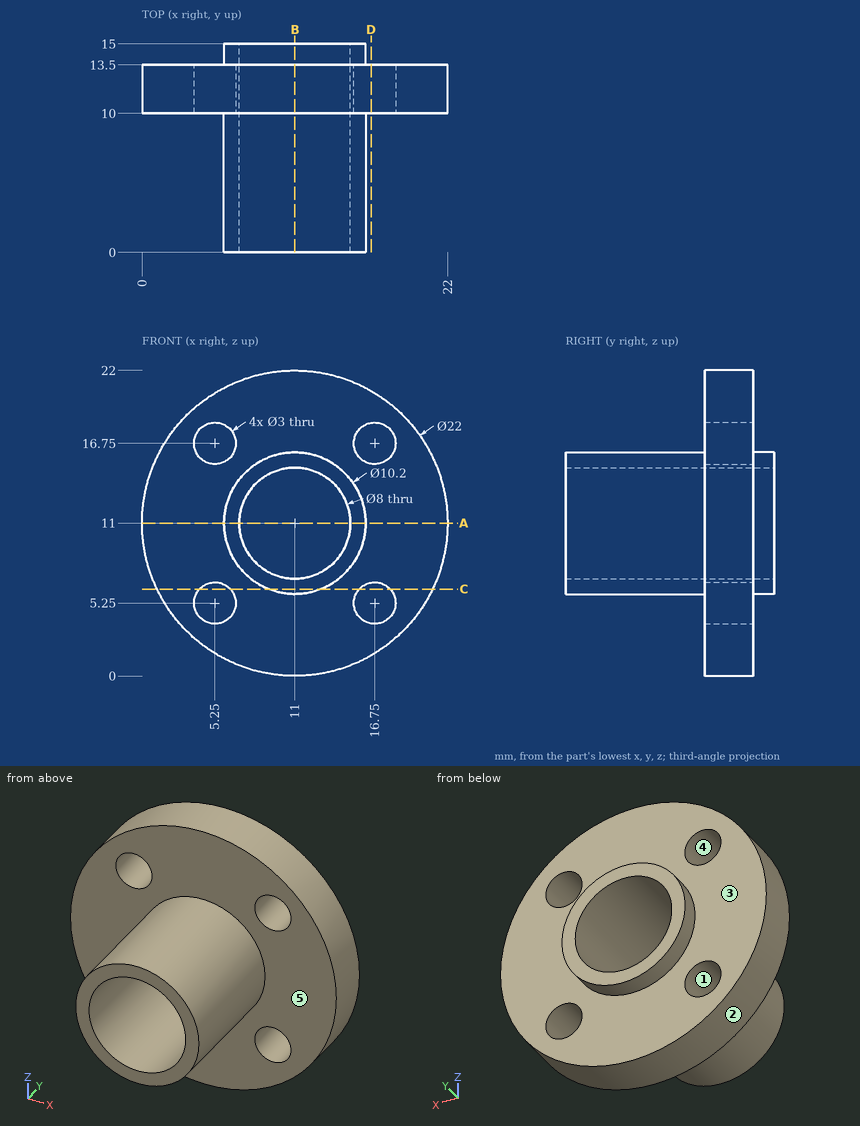
Design review of the part shown in the three views and the two pictorial views. Dimensions are in mm from the part's minimum x, y and z. A direction names the side the tool comes from. Round coordinates to 2 decimals unless told otherwise and drop trailing zeros. Order: outer loops, then holes, each group sorted by start corner. A loop starts at its lowest first (then second) coordinate and runs counter-clockwise, first axis right, second up.
Q1. We need section B-B, the plane x = 11. Give the boundary of the cut face in (y, z), plus the area to 3 significant figures.
Findings below:
outline: (0, 5.9) - (10, 5.9) - (10, 0) - (13.5, 0) - (13.5, 5.9) - (15, 5.9) - (15, 7) - (0, 7) - close; (0, 15) - (15, 15) - (15, 16.1) - (13.5, 16.1) - (13.5, 22) - (10, 22) - (10, 16.1) - (0, 16.1) - close
area: 74.3 mm2
Q2. Wall thickness on line 1 (Z direction, x = 5.25, y = 11.95); line 2 (Y direction, x = 18, z = 7.75): over which ranges is each line inside the solid? List them lowest first.
Findings below:
line 1: z = 1.62 to 3.75, 6.75 to 15.25, 18.25 to 20.38
line 2: y = 10 to 13.5
Q3. We need section A-A, the plane z = 11. Give the boundary of the cut face in (x, y).
Findings below:
outline: (0, 10) - (5.9, 10) - (5.9, 0) - (7, 0) - (7, 15) - (5.9, 15) - (5.9, 13.5) - (0, 13.5) - close; (15, 0) - (16.1, 0) - (16.1, 10) - (22, 10) - (22, 13.5) - (16.1, 13.5) - (16.1, 15) - (15, 15) - close
Q4. Machinability: for the marked faces 4 and 5, which of the approach directions +Z, -Z, +X, -X, +Y, -Y give a long, thin tool a straight path to every point of the face, cutting with its end or side? Answer none if there is none.
Findings below:
face 4: +Y, -Y
face 5: -Y
Q5. We need section D-D, the plane x = 16.5. Give the boundary of the cut face in (y, z), plus the area to 3 significant figures.
Findings below:
outline: (10, 1.47) - (13.5, 1.47) - (13.5, 3.77) - (10, 3.77) - close; (10, 6.73) - (13.5, 6.73) - (13.5, 15.27) - (10, 15.27) - close; (10, 18.23) - (13.5, 18.23) - (13.5, 20.53) - (10, 20.53) - close
area: 46.0 mm2
Q6. We need section C-C, the plane z = 6.25. Give the boundary of the cut face in (x, y).
Findings below:
outline: (1.08, 10) - (4.13, 10) - (4.13, 13.5) - (1.08, 13.5) - close; (6.37, 10) - (9.14, 10) - (9.14, 0) - (12.86, 0) - (12.86, 10) - (15.63, 10) - (15.63, 13.5) - (12.86, 13.5) - (12.86, 15) - (9.14, 15) - (9.14, 13.5) - (6.37, 13.5) - close; (17.87, 10) - (20.92, 10) - (20.92, 13.5) - (17.87, 13.5) - close
Q7. Mouldability with a two-part tool opening along X and no side actions: class the marked faces 1, 2 and 3 as pulls with the +X half, pulls with the -X half, needs draft (parallel to the pull), parting line crosses it, or undercut.
Findings below:
face 1: undercut
face 2: parting line crosses it
face 3: needs draft
Q8. Insertion check: P1, Ø1.8, axis at x = 5.25, z = 5.25, coming from the -Y side; P2, Ø6, axis at x = 8.5, y = 12, coming from the +Z side; P3, Ø5, axis at x = 16.75, z = 16.75, coming from the +Y side; P4, Ø3, axis at x = 8.5, y = 3.5, coming from the -Z side. Each pin has a flat end and moves straight along its axis. Give the tip position at first contact, or say it passes through.
Findings below:
P1: passes through
P2: stops at z = 22
P3: stops at y = 13.5
P4: stops at z = 6
